Job drawing, mm, ordinate dimensions from the low corner. One solid piece. Round coordinates to 2 decimals unless told otherwise and drop trailing zeros. Loops run counter-clockwise (first coordinate to the right, second up) from the corner with the lowest first, then second, coordinate; pieces in that order, holes last.
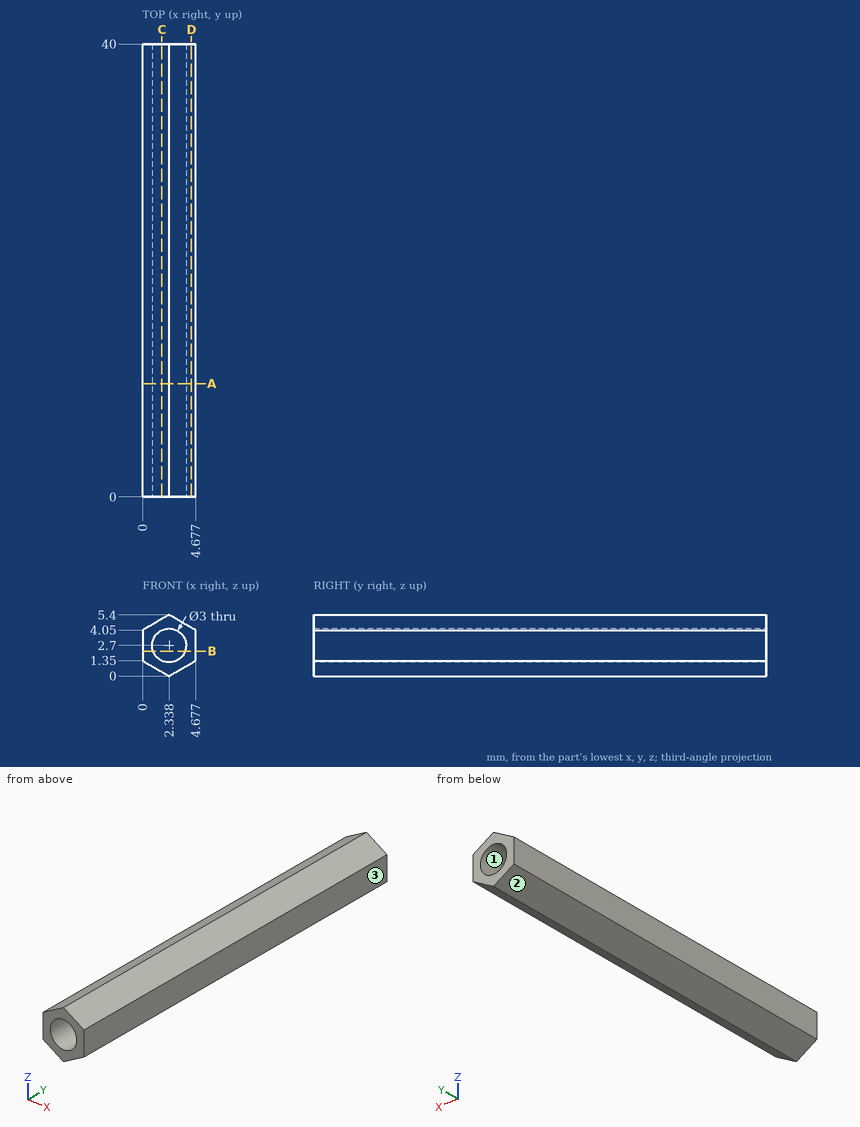
(1) Slice it at C-C on x = 1.7. List the corners of the cut face in (y, z).
Responses:
outline: (0, 0.37) - (40, 0.37) - (40, 1.34) - (0, 1.34) - close; (0, 4.06) - (40, 4.06) - (40, 5.03) - (0, 5.03) - close
(2) Pull direction X, two halves, no side cores. Call the marked faces 1, 2 and 3: +X half, -X half, draft (parallel to the pull), parting line (faces both ways), or undercut.
Responses:
face 1: undercut
face 2: -X half
face 3: +X half
(3) Slice it at B-B on z = 2.2. List the corners of the cut face in (x, y).
Responses:
outline: (0, 0) - (0.92, 0) - (0.92, 40) - (0, 40) - close; (3.75, 0) - (4.68, 0) - (4.68, 40) - (3.75, 40) - close
(4) Slice it at D-D on x = 4.3. List the corners of the cut face in (y, z).
Responses:
outline: (0, 1.13) - (40, 1.13) - (40, 4.27) - (0, 4.27) - close
(5) Probe line 1 (X direction, y = 10, z = 2.7); line 2 (Z direction, x = 1.85, y = 35); line 3 (Z direction, x = 2.5, y = 8) (1 decimal). List the from-to ranges inside material, lowest first.
Responses:
line 1: x = 0 to 0.84, 3.84 to 4.68
line 2: z = 0.28 to 1.28, 4.12 to 5.12
line 3: z = 0.1 to 1.2, 4.2 to 5.3
(6) Slice it at A-A on y = 10. List the corners of the cut face in (x, z).
Responses:
outline: (0, 1.35) - (2.34, 0) - (4.68, 1.35) - (4.68, 4.05) - (2.34, 5.4) - (0, 4.05) - close; hole circle Ø3 at (2.34, 2.7)
